Geometry check sheet. Reference: the model listing, model coordinates, mm. Round coordinates to 2 decimals unless told otherwise and drop trailing zeros. Order: outer loops, then holes, each group sorted by start corner. A loop starts at its lowest first (then second) coordinate and runs counter-clockwise, first axis right, second up.
(1) Thickness scan on L1, parallel to X at y = 11, z = 173.5; L2, parallel to X at y = 70, z = 302.5; L3, parallel to Z at x = -143.5, y = 70.5. Record the ranges inside material, lowest first.
(2) Cross-section at A-A on y = 149. Enter the section's corners in (x, z).
(3) Cross-section at D-D on z = 257.5. Enter the section's corners in (x, y), and give its area (3 significant figures).
(4) Gauge pin test, flat ends, axial feed: P1, Ø8, axis at y = 83, z = 299.5, coming from the -X side; P2, Ø5, axis at x = 28.5, y = 86, coming from the -Z side; P3, Ø3, axis at y = 128.5, z = 54.5, coming from the +X side; P4, Ø8, axis at x = -180.5, z = 230.5, coming from the +Y side. Record the tip position at first contact, or that the pin passes through.
(5) Cross-section at C-C on z = 201. Enter the section's corners in (x, y), and give its area (3 significant figures).
(6) Cross-section at B-B on x = -48. Enter the section's corners in (y, z).
from build123d import *

# Parameters (mm, degrees)
F1_DEPTH = 25.4
F2_DEPTH = 165.608


with BuildPart() as f1:
    # F0 (on Front) → F1 (new body)
    with BuildSketch(Plane.XZ):
        Polygon((28.065755, -33.692958), (78.471489, -91.832571), (57.925102, 34.130888), align=None)
        Polygon((-61.737064, 69.888532), (28.065755, -33.692958), (57.925102, 34.130888), (57.516154, 36.638021), align=None)
        Polygon((-69.187544, 88.35157), (-61.737064, 69.888532), (57.516154, 36.638021), (-270.528197, 350.663453), align=None)
    extrude(amount=F1_DEPTH)

    # F1_face (on face) → F2 (join)
    with BuildSketch(Plane(origin=(-46.516677, 0, 96.881853), x_dir=(1, 0, 0), z_dir=(0, 1, 0))):
        Polygon((104.032831, 60.243832), (124.988166, 188.714424), (-15.220387, 26.993321), (-22.670867, 8.530283), (-224.01152, -253.7816), align=None)
    extrude(amount=F2_DEPTH)


solid = f1.part
Found:
1. L1: x = -134.54 to -85.46
1. L2: x = -233.56 to -220.21
1. L3: z = 185.17 to 229.06
2. outline: (-270.53, 350.66) - (-69.19, 88.35) - (-61.74, 69.89) - (78.47, -91.83) - (57.52, 36.64) - close
3. outline: (-199.02, -25.4) - (-173.21, -25.4) - (-173.21, 165.61) - (-199.02, 165.61) - close
3. area: 4,930 mm2
4. P1: stops at x = -234.33
4. P2: stops at z = -37.08
4. P3: stops at x = 40.42
4. P4: stops at y = 165.61
5. outline: (-155.65, -25.4) - (-114.18, -25.4) - (-114.18, 165.61) - (-155.65, 165.61) - close
5. area: 7,920 mm2
6. outline: (-25.4, 54.04) - (165.61, 54.04) - (165.61, 137.64) - (-25.4, 137.64) - close
